Source: CAD feature listing. Evaluate the final solid. Frame: model axes, mm. Face numbers are marked on the shaded views. A direction names the side the tool comes from. Give positions to 0.01 mm unless a question says otherwise; leave off trailing zeros. Order: outer loops, then holes, each group sorted by start corner. A loop starts at its lowest first (then second) coordinate and runs counter-clockwise, first axis right, second up.
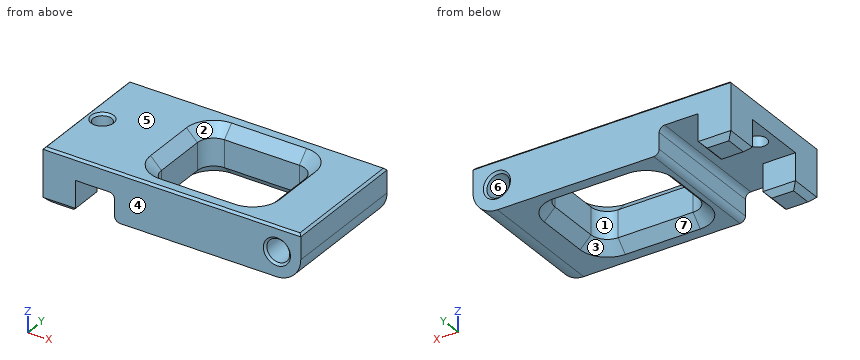
Autodesk Fusion 360 part; units mm, degrees
sketch "Sketch1" plane through (0, 0, 0) normal (0, 1, 0) x (1, 0, 0) in component "bowen_retainer"
  line L0 (-24, -4) -> (23.5, -4)
  line L1 (23.5, -4) -> (23.5, 5)
  line L2 (23.5, 5) -> (-10.809, 5)
  line L3 (-10.809, 5) -> (-10.809, 0)
  line L4 (-10.809, 0) -> (-18, 0)
  line L5 (-18, 0) -> (-18, 6)
  line L6 (-18, 6) -> (-24, 6)
  line L7 (-24, 6) -> (-24, -4)
  circle A0 centre (19.1, 0.5) radius 2.1
  line L8 (23.5, 0.5) -> (19.1, 0.5) construction
  point P0 (23.5, 0.5)
  dimension "d17" = 47.5
  dimension "d18" = 6
  dimension "d19" = 6
  dimension "d22" = 9
  dimension "d23" = 4.2
  dimension "d24" = 4.4
extrude "Extrude1" add sketch "Sketch1" along normal mid plane 24 in component "bowen_retainer"
sketch "Sketch2" plane through (0, 0, 4) normal (0, 0, 1) x (-1, 0, 0) in component "bowen_retainer"
  line L0 (-23.5, 12) -> (-23.5, -12)
  line L1 (-23.5, -12) -> (24, -12)
  line L2 (24, -12) -> (24, 12)
  line L3 (24, 12) -> (-23.5, 12)
  circle A0 centre (21, 0) radius 1.7
  line L4 (24, 12) -> (24, -12)
  line L5 (24, -12) -> (18, -12)
  line L6 (18, -12) -> (18, 12)
  line L7 (18, 12) -> (24, 12)
  line L8 (24, -12) -> (18, 12) construction
  line L9 (24, 12) -> (18, -12) construction
  line L10 (6.809, -8) -> (-13, -8)
  line L11 (-13, -8) -> (-13, 8)
  line L12 (-13, 8) -> (6.809, 8)
  line L13 (6.809, 8) -> (6.809, -8)
  line L14 (10.809, 12) -> (10.809, -12)
  line L15 (10.809, -12) -> (-23.5, -12)
  line L16 (-23.5, -12) -> (-23.5, 12)
  line L17 (-23.5, 12) -> (10.809, 12)
  point P0 (21, 0)
  dimension "d27" = 3.4
  dimension "d28" = 4
  dimension "d29" = 4
  dimension "d30" = 10.5
  dimension "d31" = 4
extrude "Extrude2" cut sketch "Sketch2" against normal through all contours A0 | L10 L11 L12 L13 in component "bowen_retainer"
sketch "Sketch3" plane through (-24, 0, 0) normal (-1, 0, 0) x (0, -1, 0) in component "bowen_retainer"
  line L0 (12, 4) -> (-12, 4)
  line L1 (-12, 4) -> (-12, -6)
  line L2 (-12, -6) -> (12, -6)
  line L3 (12, -6) -> (12, 4)
  line L4 (-6, -6) -> (6, -6)
  line L5 (6, -6) -> (6, 0)
  line L6 (6, 0) -> (-6, 0)
  line L7 (-6, 0) -> (-6, -6)
  line L8 (12, 0) -> (-12, 0)
  line L9 (-12, 0) -> (-12, -5)
  line L10 (-12, -5) -> (12, -5)
  line L11 (12, -5) -> (12, 0)
  dimension "d33" = 6
extrude "Extrude3" cut sketch "Sketch3" against normal up to surface (6 mm away) contours L5 L6 L7 L8 L10 | L2 L4 L5 L7 L10 in component "bowen_retainer"
fillet "Fillet1" radius 4.5 1 edges at (23.5, 0, -5) in component "bowen_retainer"
fillet "Fillet2" radius 3 4 edges at (-6.809, 8, -0.5) (13, 8, -0.5) (13, -8, -0.5) (-6.809, -8, -0.5) in component "bowen_retainer"
chamfer "Chamfer1" distance 2 angle 45 16 edges at (-5.9304, 7.1213, 4) (-6.809, 0, 4) (-5.9304, -7.1213, 4) (3.0955, -8, 4) (12.1213, -7.1213, 4) (13, 0, 4) (12.1213, 7.1213, 4) (3.0955, 8, 4) (-6.809, 0, -5) (-5.9304, -7.1213, -5) (3.0955, -8, -5) (12.1213, -7.1213, -5) (13, 0, -5) (12.1213, 7.1213, -5) (3.0955, 8, -5) (-5.9304, 7.1213, -5) in component "bowen_retainer"
fillet "Fillet3" radius 1 2 edges at (-10.809, 0, 0) (-10.809, 0, -5) in component "bowen_retainer"
chamfer "Chamfer2" distance 1 angle 45 2 edges at (-24, 9, -6) (-21, 12, -6) 2 faces at (-20, 8, -6) (-20, -8, -6) in component "bowen_retainer"
chamfer "Chamfer3" distance 0.4 angle 45 7 edges at (-19.415, -0.6147, 4) (17.1421, -12, 0.2594) (17.1421, 12, -1.2594) (-0.25, 12, 4) (23.5, 0, 4) (-0.25, -12, 4) (-24, 0, 4) in component "bowen_retainer"
component "bowen_retainer" placed x (1, 0, 0) y (0, 1, 0) z (0, 0, 1) at (0, 0, 0)
equation "ptfe_tube_od = 4 mm"
equation "tolerance = 0.2 mm"
equation "extrusion_width = 20 mm"
equation "width = 24 mm"
equation "length = 47.5 mm"
equation "arm_width = 4 mm"
equation "extrusion_slot_width = 6 mm"
equation "d17 = length"
equation "d18 = extrusion_slot_width"
equation "d19 = extrusion_slot_depth"
equation "extrusion_slot_depth = 6 mm"
equation "depth = 9 mm"
equation "d22 = depth"
equation "d23 = ptfe_tube_od + tolerance"
equation "d25 = width"
equation "d28 = arm_width"
equation "d29 = arm_width"
equation "d33 = extrusion_slot_depth"
1) Section query A-A, the plane y = 0. Return the cut outline in (x, z).
Report:
outline: (-24, 0) - (-22.7, 0) - (-22.7, 3.6) - (-23.1, 4) - (-23.6, 4) - (-24, 3.6) - close; (-19.3, 0) - (-11.81, 0) arc R1 cw to (-10.81, -1) - (-10.81, -4) arc R1 ccw to (-9.81, -5) - (-8.81, -5) - (-6.81, -3) - (-6.81, 2) - (-8.81, 4) - (-18.9, 4) - (-19.3, 3.6) - close; (13, -3) - (15, -5) - (19, -5) arc R4.5 ccw to (23.5, -0.5) - (23.5, 3.6) - (23.1, 4) - (15, 4) - (13, 2) - close; hole circle Ø4.2 at (19.1, -0.5)
2) Draft query along Z for the marked faces 4, 5, 6 and 7. Return one class per face: +Z half, -Z half, draft (parallel to the pull), parting line (faces both ways), or undercut.
Report:
face 4: draft
face 5: +Z half
face 6: undercut
face 7: -Z half
3) Reachability of the marked faces 1, 2 and 3 from +Z, -Z, +X, -X, +Y, -Y: full face, straight path, thin tool, end or side. Return the list, or none.
Report:
face 1: +Z, -Z
face 2: +Z
face 3: -Z
4) Material intervals for L1, parallel to Z at x = 19.1, y = -1.25; L2, parallel to X at y = 0, z = 2.3; L3, parallel to X at y = 1, z = 3.5, sorted ascending.
Report:
L1: z = -5 to -2.6, 1.6 to 4
L2: x = -24 to -22.7, -19.3 to -7.11, 13.3 to 23.5
L3: x = -24 to -22.37, -19.63 to -8.31, 14.5 to 23.5
5) Section query B-B, the plane x = -21. Return the cut outline in (y, z), and give its area (3 significant figures).
Report:
outline: (-12, -5) - (-11, -6) - (-7, -6) - (-6, -5) - (-6, 0) - (-1.7, 0) - (-1.7, 3.6) - (-2.1, 4) - (-11.6, 4) - (-12, 3.6) - close; (1.7, 0) - (6, 0) - (6, -5) - (7, -6) - (11, -6) - (12, -5) - (12, 3.6) - (11.6, 4) - (2.1, 4) - (1.7, 3.6) - close
area: 152 mm2
6) Section query C-C, the plane y = -10.5. Return the cut outline in (x, z), and give its area (3 significant figures).
Report:
outline: (-24, -5) - (-23, -6) - (-19, -6) - (-18, -5) - (-18, 0) - (-11.81, 0) arc R1 cw to (-10.81, -1) - (-10.81, -4) arc R1 ccw to (-9.81, -5) - (19, -5) arc R4.5 ccw to (23.5, -0.5) - (23.5, 3.6) - (23.1, 4) - (-23.6, 4) - (-24, 3.6) - close; hole circle Ø4.2 at (19.1, -0.5)
area: 378 mm2
7) Section query D-D, the plane x = 7.5. Return the cut outline in (y, z), and give its area (3 significant figures).
Report:
outline: (-12, -5) - (-10, -5) - (-8, -3) - (-8, 2) - (-10, 4) - (-11.6, 4) - (-12, 3.6) - close; (8, -3) - (10, -5) - (12, -5) - (12, 3.6) - (11.6, 4) - (10, 4) - (8, 2) - close
area: 63.8 mm2
8) Pin query (flat end, axial travel): pin 1 (2.5 mm diameter, centred on y = -8, z = -3, fed in from +X); pin 2 (6 mm diameter, centred on x = 15, y = -8.5, fed in from -Z); pin 3 (4 mm diameter, centred on x = 19.1, z = -0.5, fed in from +Y); pin 4 (5 mm diameter, centred on y = 3, z = -3.5, fed in from -X). Return the tip coordinate at first contact, or that it passes through.
Report:
pin 1: stops at x = 23.32
pin 2: stops at z = -5
pin 3: passes through
pin 4: stops at x = -10.81
